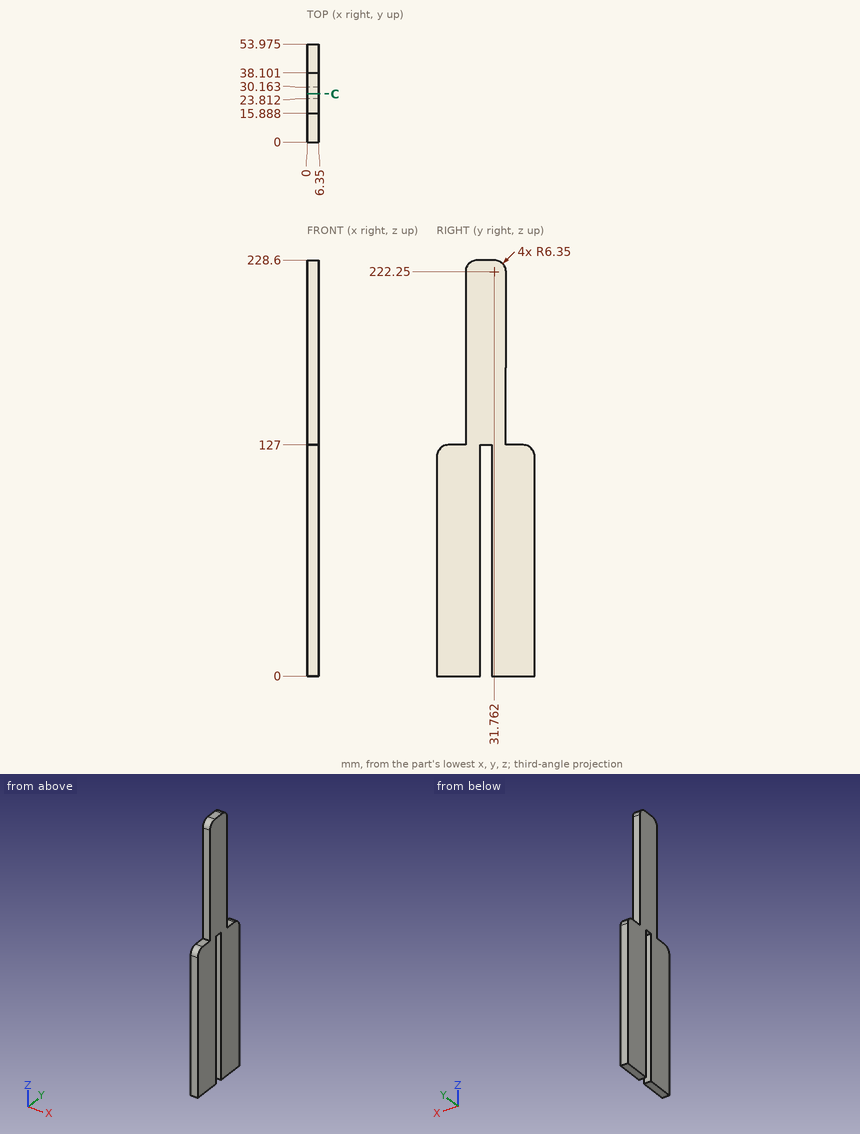
Print and shaded views of the part. All mm, measured from the part's lowest x, y and z. Give positions to 0.01 mm unless a question says otherwise; leave off trailing zeros. Order: outer loops, then holes, each group sorted by start corner. A loop starts at its lowest first (then second) coordinate and runs counter-clockwise, first axis right, second up. Notation, with made-up numbers: (-7, 12) - (34, 12) arc R18 ccw to (34, 35) - close; hole circle Ø7 at (32.5, -3.5). An arc over 180 degrees is marked (long way). One line per item, written item: value.
Item 1: Slice it at C-C (y = 26.5). List the corners of the cut face in (x, z).
Response values:
outline: (0, 127) - (6.35, 127) - (6.35, 228.6) - (0, 228.6) - close
Item 2: Pin check, flat tips, straight feed: pin 1 Ø3 at (x, y) = (3.5, 26) entering from -Z; pin 2 Ø3 at (x, z) = (4, 157) entering from +Y (1 decimal); pin 3 Ø8 at (y, z) = (10, 194.5) entering from +X; pin 4 Ø3 at (x, y) = (2, 11) entering from +Z. Stop position of each tip, or through.
Response values:
pin 1: z = 127
pin 2: y = 38.1
pin 3: through
pin 4: z = 127
Item 3: Wall check: line 1 (Y direction, x = 4, z = 39.5) (1 decimal); line 2 (Z direction, x = 4, y = 40); line 3 (Z direction, x = 5, y = 21.5). Give the ranges that are in metal, low to high.
Response values:
line 1: 0 to 23.8, 30.2 to 54
line 2: 0 to 127
line 3: 0 to 228.56
